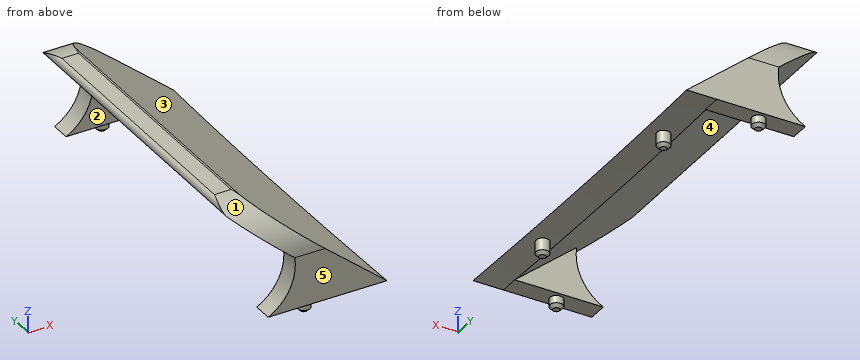
from build123d import *

# Parameters (mm, degrees)
F1_DEPTH  = 22.225
F3_DEPTH  = 14.199989
F4_R      = 311.546875
F5_DEPTH  = 38.1
F7_DEPTH  = 2.38125
F9_R      = 0.79375
F10_DEPTH = 1.27
F11_SIZE  = 0.381


with BuildPart() as f1:
    # F0 (on Front) → F1 (new body, symmetric)
    with BuildSketch(Plane.XZ):
        with BuildLine():
            Line((0, 0), (3.704567, 0))
            Line((3.704567, 0), (-11.281316, 12.574649))
            ThreePointArc((-11.281316, 12.574649), (-11.442464, 12.667688), (-11.625715, 12.7))
            Line((-11.625715, 12.7), (-13.663198, 12.7))
            ThreePointArc((-13.663198, 12.7), (-14.166677, 12.347461), (-14.007598, 11.75377))
            Line((-14.007598, 11.75377), (0, 0))
        make_face()
    extrude(amount=F1_DEPTH, both=True)

    # F2 (on Right) → F3 (cut, through all)
    with BuildSketch(Plane.YZ):
        with BuildLine():
            ThreePointArc((-22.225, 6.35), (-20.365128, 10.840128), (-15.875, 12.7))
            Line((-15.875, 12.7), (-25.184002, 17.701721))
            Line((-25.184002, 17.701721), (-26.87986, 8.657143))
            Line((-26.87986, 8.657143), (-22.225, 6.35))
        make_face()
        with BuildLine():
            Line((22.225, 6.35), (26.87986, 8.657143))
            Line((26.87986, 8.657143), (25.184002, 17.701721))
            Line((25.184002, 17.701721), (15.875, 12.7))
            ThreePointArc((15.875, 12.7), (20.365128, 10.840128), (22.225, 6.35))
        make_face()
    extrude(amount=-F3_DEPTH, mode=Mode.SUBTRACT)

    # F4 (on Right) → F5 (cut, symmetric)
    with BuildSketch(Plane.YZ):
        with Locations((0, -310.753125)):
            Circle(F4_R)
    extrude(amount=F5_DEPTH, both=True, mode=Mode.SUBTRACT)

    # F6 (on face) → F7 (join)
    with BuildSketch(Plane.XZ.offset(22.225)):
        with BuildLine():
            Line((-10.819531, 0), (0, 0))
            Line((0, 0), (-7.567635, 6.35))
            ThreePointArc((-7.567635, 6.35), (-8.1783, 2.655064), (-10.819531, 0))
        make_face()
    extrude(amount=-F7_DEPTH)



with BuildPart() as f8_1:
    # F8: instance of F1
    add(f1.part.mirror(Plane.XZ))


with BuildPart() as f1_1:
    add(f1.part)

    add(f8_1.part)  # F10 merges F8_1
    # F9 (on face) → F10 (join, symmetric)
    with BuildSketch(Plane(origin=(0, 0, 0), x_dir=(1, 0, 0), z_dir=(0, 0, -1))):
        with Locations((-5.779071, 21.034375)):
            Circle(F9_R)
        with Locations((0.871276, 12.592022)):
            Circle(F9_R)
        with Locations((0.871276, -12.592022)):
            Circle(F9_R)
        with Locations((-5.779071, -21.034375)):
            Circle(F9_R)
    extrude(amount=F10_DEPTH, both=True)

    # F11
    f11_edges = [f1_1.edges().sort_by_distance(p)[0] for p in [
        (0.077526, -12.592022, -1.27),
        (-6.572821, -21.034375, -1.27),
        (0.077526, 12.592022, -1.27),
        (-6.572821, 21.034375, -1.27),
    ]]
    chamfer(f11_edges, length=F11_SIZE)


solid = f1_1.part
Source: CAD feature listing. Evaluate the final solid. Frame: model axes, mm. Face numbers are marked on the shaded views. A direction names the side the tool comes from. Round coordinates to 2 decimals unless told otherwise and drop trailing zeros. Write each loop counter-clockwise with the first axis right and the second up, starting at its lowest first coordinate (ties: lowest second). Pieces come first, ordered by that corner, then holes. Notation, with made-up numbers: M 26.5,49.25 L 65.5,49.25 A12 cw 65.5,68.25 Z; hole C -39.5,60 d1. An arc over 180 degrees is marked long. One line per item, written item: value. Start each with the question number.
Item 1: Section query B-B (y = -1). Return the cut outline in (x, z).
Item 2: Section query C-C (z = 2.5). Return the cut outline in (x, y) (3 decimals).
Item 3: Section query D-D (y = 3.5). Return the cut outline in (x, z).
Item 4: Set-up query: the marked faces 1 and 2. Return all of +Z, -Z, +X, -X, +Y, -Y with unobstructed straight access to the full face (end or side cutting, diameter ignored); none if empty.
Item 5: Pin query (flat end, axial travel): pin 1 (2.5 mm diameter, centred on x = -7.5, y = -21, fed in from -Z); pin 2 (5 mm diameter, centred on x = -3, y = -15.5, fed in from -Z); pin 3 (8 mm diameter, centred on x = 0.5, y = 4, fed in from +Z); pin 4 (2 mm diameter, centred on x = -9.5, z = 2.5, fed in from +Y). Return the tip coordinate at first contact, or that it passes through.
Item 6: Section query A-A (x = -2.5). Return the cut outline in (y, z) (3 decimals).
Item 7: Mould query, pull axis Y, two halves, no side actions, for the marked faces 3, 4 and 5. Classes: pulls with the +Y half, pulls with the -Y half, needs draft (parallel to the pull), parting line crosses it, or undercut.
Item 8: Ray query, L1, parallel to Y at x = -2.5, z = 1.5 (3 decimals); L2, parallel to Z at x = -13, y = -11.5; L3, parallel to X at y = 2, z = 2.5. Return the intervals inside material, ascending. Write a range as from..to.
Result set:
1. outline: M -14.01,11.75 L -0.94,0.79 L 2.76,0.79 L -11.28,12.57 A0.54 ccw -11.63,12.7 L -13.66,12.7 A0.54 ccw Z
2. outline: M -8.261,-22.225 L 0.725,-22.225 L 0.725,22.225 L -8.261,22.225 L -8.261,19.844 L -2.979,19.844 L -2.979,-19.844 L -8.261,-19.844 Z
3. outline: M -14.01,11.75 L -0.92,0.77 L 2.78,0.77 L -11.28,12.57 A0.54 ccw -11.63,12.7 L -13.66,12.7 A0.54 ccw Z
4. face 1: +Z, +X, -X, -Y
4. face 2: -Z, -X
5. pin 1: stops at z = -1.21
5. pin 2: stops at z = 0.42
5. pin 3: stops at z = 6.05
5. pin 4: passes through
6. outline: M -22.225,0 L -19.844,0 L -19.844,2.098 L 19.844,2.098 L 19.844,0 L 22.225,0 L 22.225,5.206 L -22.225,5.206 Z
7. face 3: needs draft
7. face 4: undercut
7. face 5: pulls with the -Y half
8. L1: y = -22.225..-19.844, 19.844..22.225
8. L2: z = 10.91..12.7
8. L3: x = -2.98..0.73
